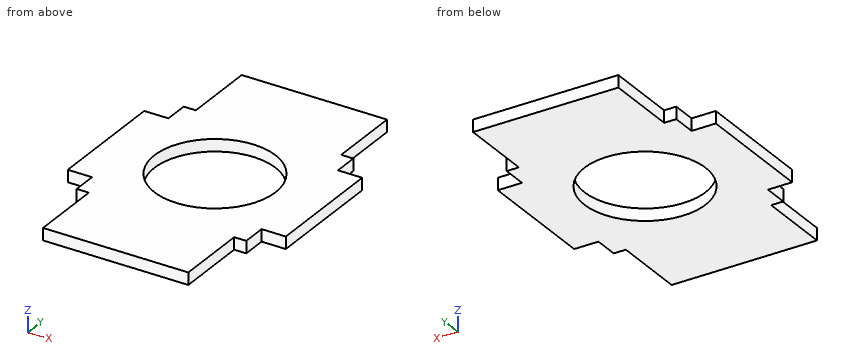
from build123d import *

# Parameters (mm, degrees)
SKETCH1_R           = 15.875
BOSS_EXTRUDE1_DEPTH = 3.175


with BuildPart() as part:
    # Sketch1 → Boss-Extrude1 (new body)
    with BuildSketch(Plane.XY):
        Polygon((-0.558515458, 289.07227709), (37.541484542, 289.07227709), (37.541484542, 308.12227709), (40.716484541, 308.12227709), (40.716484541, 314.47227709), (47.06648454, 314.47227709), (47.06648454, 346.22227709), (40.716484541, 346.22227709), (40.716484541, 352.57227709), (37.541484542, 352.57227709), (37.541484542, 371.62227709), (-0.558515458, 371.62227709), (-0.558515458, 352.57227709), (-3.733515459, 352.57227709), (-3.733515459, 346.22227709), (-10.083515458, 346.22227709), (-10.083515458, 314.47227709), (-3.733515459, 314.47227709), (-3.733515459, 308.12227709), (-0.558515458, 308.12227709), align=None)
        with Locations((18.491484542, 330.34727709)):
            Circle(SKETCH1_R, mode=Mode.SUBTRACT)
    extrude(amount=-BOSS_EXTRUDE1_DEPTH)


solid = part.part
Geometry check sheet. Reference: the model listing, model coordinates, mm. Give positions to 0.01 mm unless a question says otherwise; leave off trailing zeros. Order: outer loops, then holes, each group sorted by start corner. A loop starts at its lowest first (then second) coordinate and runs counter-clockwise, first axis right, second up. Notation, with made-up numbers: (1, 20.5) - (59, 20.5) arc R25 ccw to (59, 44.5) - close; hole circle Ø4 at (57, 44). An arc over 180 degrees is marked (long way). Use one line per item in the form item = value.
1) Sectioned sample at B-B (x = 5). Record the boundary of the cut face in (y, z) (3 decimals), and give its area (3 significant figures).
Working result:
outline = (289.072, -3.175) - (321.981, -3.175) - (321.981, 0) - (289.072, 0) - close; (338.714, -3.175) - (371.622, -3.175) - (371.622, 0) - (338.714, 0) - close
area = 209 mm^2
2) Sectioned sample at A-A (y = 341.5). Record the boundary of the cut face in (x, z) (3 decimals).
Working result:
outline = (-10.084, -3.175) - (7.194, -3.175) - (7.194, 0) - (-10.084, 0) - close; (29.789, -3.175) - (47.066, -3.175) - (47.066, 0) - (29.789, 0) - close
3) Sectioned sample at C-C (z = -2.25). Record the boundary of the cut face in (x, y) (3 decimals).
Working result:
outline = (-10.084, 314.472) - (-3.734, 314.472) - (-3.734, 308.122) - (-0.559, 308.122) - (-0.559, 289.072) - (37.541, 289.072) - (37.541, 308.122) - (40.716, 308.122) - (40.716, 314.472) - (47.066, 314.472) - (47.066, 346.222) - (40.716, 346.222) - (40.716, 352.572) - (37.541, 352.572) - (37.541, 371.622) - (-0.559, 371.622) - (-0.559, 352.572) - (-3.734, 352.572) - (-3.734, 346.222) - (-10.084, 346.222) - close; hole circle Ø31.75 at (18.491, 330.347)
4) Material ranges on probe 1 along Y at (x, z) = (18, -2); probe 2 along X at (y, z) = (294, -0.85); probe 3 along X at (y, z) = (324, -1.55), recorded low to high. Write a range as from..to.
Working result:
probe_1 = 289.07..314.48, 346.21..371.62
probe_2 = -0.56..37.54
probe_3 = -10.08..3.94, 33.04..47.07
5) Depth check by flat-ended pin: pin 1 Ø1.6 at (x, z) = (39, -2.5) entering from +Y; pin 2 Ø1.6 at (y, z) = (350.5, -1.5) entering from -X; pin 3 Ø1 at (x, z) = (-2.5, -1.5) entering from -Y. Enter the tip coordinate at first touch or a pass-through.
Working result:
pin_1 = 352.57
pin_2 = -3.73
pin_3 = 308.12
6) Sectioned sample at D-D (x = -1.5). Record the boundary of the cut face in (y, z) (3 decimals).
Working result:
outline = (308.122, -3.175) - (352.572, -3.175) - (352.572, 0) - (308.122, 0) - close
